Part print with two shaded views. Sizes in mm from the minimum x, y, z corner. A direction names the side the tool comes from. Round coordinates to 2 decimals unless told otherwise and drop trailing zeros. Loops run counter-clockwise (first coordinate to the right, second up) from the corner with the lowest first, then second, coordinate; pieces in that order, holes last.
(1) Cut at C-C on z = 14. List the corners of the cut face in (x, y), then the cut area to 3 significant figures.
(2) Cut at D-D on z = 3.25. List the corners of the cut face in (x, y), then the cut area to 3 significant figures.
(3) Cut at A-A on x = 59.5. List the corners of the cut face in (y, z).
(4) Mould opens along X. For the marked faces 1, 2, 3 and 4 say: +X half, -X half, draft (parallel to the pull), parting line (faces both ways), or undercut.
(5) Probe probe 1 along X at (y, z) = (1.15, 14); probe 2 along Z at (x, y) = (59.5, 0.5); probe 3 along X at (y, z) = (16.25, 17.75). List the from-to ranges inside material, lowest first.
(6) Tool access for the marked faces 5, 6, 7 and 8: list every direction of +Z, -Z, +X, -X, +Y, -Y with a clear straight run to the whole face (end or side of a thin tool).
(7) Cut at B-B on y = 7. List the corners of the cut face in (x, z), then the cut area to 3 significant figures.
(8) Flat gauge pins, fed straight in: pin 1 (3 mm diameter, centred on y = 5, z = 5, fed in from -X); pin 2 (1 mm diameter, centred on x = 8.5, z = 2.5, fed in from +Y); pin 3 (6 mm diameter, centred on x = 30, z = 13, fed in from -Y). Where does each tip first touch, or does it go through?
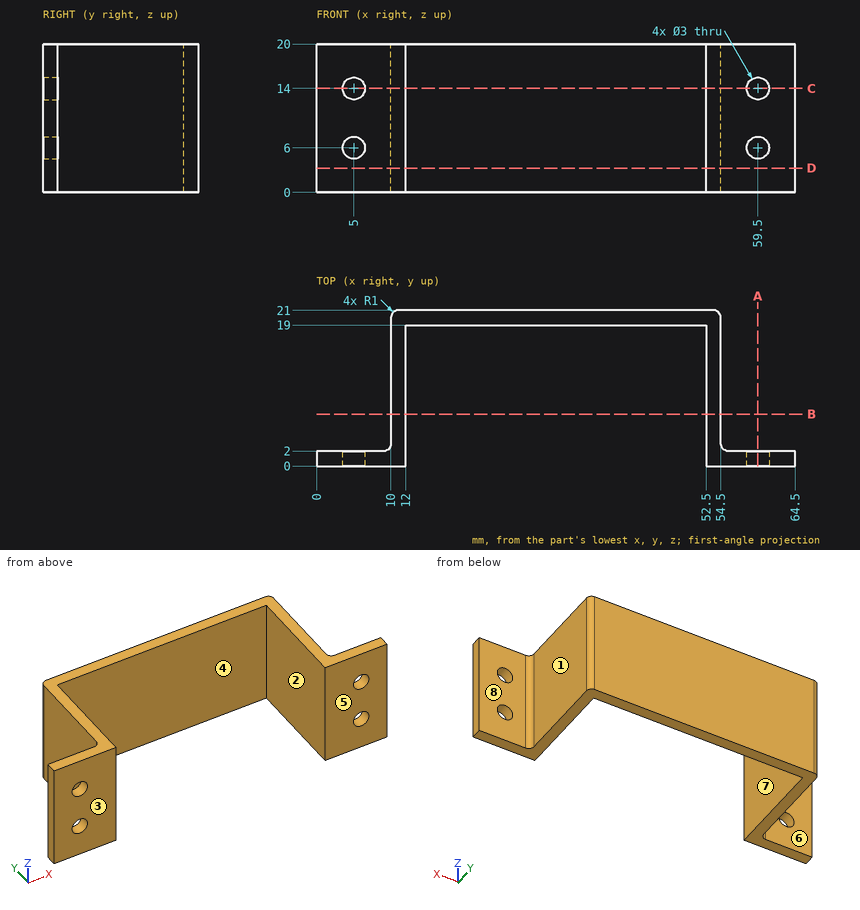
Final values:
1. outline: (0, 0) - (3.5, 0) - (3.5, 2) - (0, 2) - close; (6.5, 0) - (12, 0) - (12, 19) - (52.5, 19) - (52.5, 0) - (58, 0) - (58, 2) - (55.5, 2) arc R1 cw to (54.5, 3) - (54.5, 20) arc R1 ccw to (53.5, 21) - (11, 21) arc R1 ccw to (10, 20) - (10, 3) arc R1 cw to (9, 2) - (6.5, 2) - close; (61, 0) - (64.5, 0) - (64.5, 2) - (61, 2) - close
1. area: 193 mm2
2. outline: (0, 0) - (12, 0) - (12, 19) - (52.5, 19) - (52.5, 0) - (64.5, 0) - (64.5, 2) - (55.5, 2) arc R1 cw to (54.5, 3) - (54.5, 20) arc R1 ccw to (53.5, 21) - (11, 21) arc R1 ccw to (10, 20) - (10, 3) arc R1 cw to (9, 2) - (0, 2) - close
2. area: 205 mm2
3. outline: (0, 0) - (2, 0) - (2, 4.5) - (0, 4.5) - close; (0, 7.5) - (2, 7.5) - (2, 12.5) - (0, 12.5) - close; (0, 15.5) - (2, 15.5) - (2, 20) - (0, 20) - close
4. face 1: +X half
4. face 2: undercut
4. face 3: draft
4. face 4: undercut
5. probe 1: x = 0 to 3.5, 6.5 to 12, 52.5 to 58, 61 to 64.5
5. probe 2: z = 0 to 4.5, 7.5 to 12.5, 15.5 to 20
5. probe 3: x = 10 to 12, 52.5 to 54.5
6. face 5: +Z, -Z, +X, -X, -Y
6. face 6: +Z, -Z, -X, +Y
6. face 7: +Z, -Z, -Y
6. face 8: +Z, -Z, +X, +Y
7. outline: (10, 0) - (12, 0) - (12, 20) - (10, 20) - close; (52.5, 0) - (54.5, 0) - (54.5, 20) - (52.5, 20) - close
7. area: 80.0 mm2
8. pin 1: stops at x = 10
8. pin 2: stops at y = 2
8. pin 3: stops at y = 19
